Work out the finished part from the listing and answer in its coordinate system (mm). A direction names the side the tool comes from. Round coordinates to 2 decimals unless told otherwise and drop trailing zeros. Write each loop counter-clockwise with the first axis right and the second up, starting at its lowest first coordinate (ties: lowest second). Pieces come first, ordered by that corner, then holes. Notation, with made-up numbers: (46, 32.25) -> (105, 32.25) arc R16 cw to (105, 40.25) -> close; hole circle Ø9 at (-35, 6). An arc over 180 degrees is marked (long way). One line per item, written item: value.
```python
from build123d import *

# Parameters (mm, degrees)
SKETCH_1_W          = 150
SKETCH_1_H          = 28
EXTRUDE_1_DEPTH     = 4
CUT_EXTRUDE_1_DEPTH = 77.40026178
SKETCH_4_R          = 1.5
CUT_EXTRUDE_2_DEPTH = 77.40026178
EXTRUDE_START       = -4
SKETCH_5_W          = 18
SKETCH_5_H          = 35
SKETCH_5_R          = 1
EXTRUDE_3_DEPTH     = 4
SKETCH_7_W          = 6
SKETCH_7_H          = 6
SKETCH_7_R          = 1.5
EXTRUDE_4_DEPTH     = 4
SKETCH_3_W          = 16
SKETCH_3_H          = 10
SKETCH_3_H_2        = 11
SKETCH_3_R          = 1.5
EXTRUDE_2_DEPTH     = 4
FILLET_1_R          = 5


with BuildPart() as part:
    # Эскиз1 → Бобышка-Вытянуть1 (new body)
    with BuildSketch(Plane.XY):
        Rectangle(SKETCH_1_W, SKETCH_1_H)
    extrude(amount=EXTRUDE_1_DEPTH)

    # Эскиз2 → Вырез-Вытянуть1 (cut, through all)
    with BuildSketch(Plane.XY.offset(4)):
        with BuildLine():
            Line((-52.251534571, 1.5), (52.251534571, 1.5))
            ThreePointArc((52.251534571, 1.5), (53.751534571, 0), (52.251534571, -1.5))
            Line((52.251534571, -1.5), (-52.251534571, -1.5))
            ThreePointArc((-52.251534571, -1.5), (-53.751534571, 0), (-52.251534571, 1.5))
        make_face()
    extrude(amount=-CUT_EXTRUDE_1_DEPTH, mode=Mode.SUBTRACT)

    # Эскиз4 → Вырез-Вытянуть2 (cut, through all)
    with BuildSketch(Plane.XY.offset(4)):
        with Locations((13.699103215, -11.003765504)):
            Circle(SKETCH_4_R)
        with Locations((63.699103215, -11.003765504)):
            Circle(SKETCH_4_R)
        with Locations(Location((63.699103215, 11.003765504, 0), (0, 0, 180))):
            Circle(SKETCH_4_R)
        with Locations(Location((13.699103215, 11.003765504, 0), (0, 0, 180))):
            Circle(SKETCH_4_R)
    extrude(amount=-CUT_EXTRUDE_2_DEPTH, mode=Mode.SUBTRACT)

    # Эскиз5 → Бобышка-Вытянуть3 (add)
    with BuildSketch(Plane(origin=(0, 0, 0), x_dir=(-1, 0, 0), z_dir=(0, 0, -1)).offset(EXTRUDE_START)):
        with Locations((-84, 4.714716343)):
            Rectangle(SKETCH_5_W, SKETCH_5_H)
        with Locations((-84, -8.575)):
            Circle(SKETCH_5_R, mode=Mode.SUBTRACT)
        with BuildLine():
            ThreePointArc((-81.041084454, 5.505208333), (-78.635499923, 3.206967246), (-77.75, 0))
            ThreePointArc((-77.75, 0), (-87.206967246, -5.364500077), (-86.958915546, 5.505208333))
            ThreePointArc((-86.958915546, 5.505208333), (-84.248247218, 8.989711243), (-81, 6))
            ThreePointArc((-81, 6), (-81.010288757, 5.751752782), (-81.041084454, 5.505208333))
        make_face(mode=Mode.SUBTRACT)
        with Locations((-84, 18.825)):
            Circle(SKETCH_5_R, mode=Mode.SUBTRACT)
    extrude(amount=EXTRUDE_3_DEPTH)

    # Эскиз7 → Бобышка-Вытянуть4 (add)
    with BuildSketch(Plane.XY.offset(4)):
        with Locations((72, 19.214716343)):
            Rectangle(SKETCH_7_W, SKETCH_7_H)
        with Locations((72, 19.214716343)):
            Circle(SKETCH_7_R, mode=Mode.SUBTRACT)
    extrude(amount=-EXTRUDE_4_DEPTH)

    # Эскиз3 → Бобышка-Вытянуть2 (add)
    # profile 1 of 4: a face of its own
    with BuildSketch(Plane.XY.offset(4)):
        with Locations((-15, 9)):
            Rectangle(SKETCH_3_W, SKETCH_3_H)
    # profile 2 of 4: a face of its own
    with BuildSketch(Plane.XY.offset(4)):
        with Locations((-15, 19.5)):
            Rectangle(SKETCH_3_W, SKETCH_3_H_2)
        with Locations((-15, 19.5)):
            Circle(SKETCH_3_R, mode=Mode.SUBTRACT)
    # profile 3 of 4: a face of its own
    with BuildSketch(Plane.XY.offset(4)):
        with Locations((-15, -9)):
            Rectangle(SKETCH_3_W, SKETCH_3_H)
    # profile 4 of 4: a face of its own
    with BuildSketch(Plane.XY.offset(4)):
        with Locations((-15, -19.5)):
            Rectangle(SKETCH_3_W, SKETCH_3_H_2)
        with Locations((-15, -19.5)):
            Circle(SKETCH_3_R, mode=Mode.SUBTRACT)
    extrude(amount=-EXTRUDE_2_DEPTH)

    # Скругление1
    fillet_1_edges = [part.edges().sort_by_distance(p)[0] for p in [
        (-23, -25, 2),
        (-7, -25, 2),
        (-7, 25, 2),
        (-23, 25, 2),
    ]]
    fillet(fillet_1_edges, radius=FILLET_1_R)


solid = part.part
```
(1) Flat-ended cylindrical pins translate along their axes: pin 1 Ø2 at (x, z) = (31, 3) entering from -Y; pin 2 Ø1.2 at (x, z) = (79.5, 2) entering from -Y. Find the tip coordinate at first contact, or state that the pin passes through.
Reported:
pin 1: stops at y = -14
pin 2: stops at y = -12.79
(2) Find section D-D on z = 2.75. Give the number of separate pieces and of enclosed holes in the cut face, plus the area to 3 significant figures.
Reported:
separate pieces: 1
enclosed holes: 11
area: 4,680 mm2
(3) A tool of negligible diameter and unlimited length cuts with its end or side. For faces 1 (the face through (8, 6, 4)), 2 (the face through (1, -1.5, 2)), 3 (the face through (-9, 24, 2)), 4 (the face through (-49, 14, 2)), 5 (the face through (84, -12.785, 2)), from which of +Z, -Z, +X, -X, +Y, -Y can it reach the whole face along a straight path? Write none if from no direction.
Reported:
face 1: +Z, +X, -X, +Y, -Y
face 2: +Z, -Z
face 3: +Z, -Z, +Y
face 4: +Z, -Z, -X, +Y
face 5: +Z, -Z, +X, -Y
(4) Find section C-C on x = -58. Give the vertices of the cut face in (y, z).
Reported:
outline: (-14, 0) -> (14, 0) -> (14, 4) -> (-14, 4) -> close
(5) Consider probe 1 along X at (y, z) = (11, 2.75); probe 2 along Y at (x, z) = (-15, 2.4); probe 3 along Y at (x, z) = (84, 2.15) (3 decimals). Determine where each line is inside the solid, lowest interval first.
Reported:
probe 1: x = -75 to 12.2, 15.2 to 62.2, 65.2 to 93
probe 2: y = -25 to -21, -18 to -1.5, 1.5 to 18, 21 to 25
probe 3: y = -12.785 to -9.575, -7.575 to -6.25, 9 to 17.825, 19.825 to 22.215
(6) Find section A-A on x = 44. Give the vertices of the cut face in (y, z).
Reported:
outline: (-14, 0) -> (-1.5, 0) -> (-1.5, 4) -> (-14, 4) -> close; (1.5, 0) -> (14, 0) -> (14, 4) -> (1.5, 4) -> close
(7) For a pull along Y with two mould halves and no side action, classify faces 6 (the face through (15.198, 10.938, 2.028)), 7 (the face through (93, 4, 2)), 8 (the face through (-15, -25, 2)) as pulls with the +Y half, pulls with the -Y half, needs draft (parallel to the pull), parting line crosses it, or undercut.
Reported:
face 6: undercut
face 7: needs draft
face 8: pulls with the -Y half
(8) Find section B-B on x = -15. Give the vertices of the cut face in (y, z), plus the area to 3 significant figures.
Reported:
outline: (-25, 0) -> (-21, 0) -> (-21, 4) -> (-25, 4) -> close; (-18, 0) -> (-1.5, 0) -> (-1.5, 4) -> (-18, 4) -> close; (1.5, 0) -> (18, 0) -> (18, 4) -> (1.5, 4) -> close; (21, 0) -> (25, 0) -> (25, 4) -> (21, 4) -> close
area: 164 mm2
